Design review of the part built by this model. Coordinates are the model's own, in mm. A direction names the side the tool comes from. Give positions to 0.01 mm unless a question says otherwise; leave off trailing zeros. Loops run counter-clockwise (first coordinate to the right, second up) from the corner with the lowest first, then second, coordinate; pieces in that order, holes last. Notation, with made-up numbers: (70.25, -30.75) - (125.25, -30.75) arc R24 cw to (125.25, -11.75) - close; hole circle Ø6 at (53.25, 10). An arc over 180 degrees is marked (long way). Put each result on its own line as item: value. Start each with the question number.
```python
from build123d import *

# Parameters (mm, degrees)
F0_W     = 4
F0_H     = 4
F1_DEPTH = 55
F2_R     = 2
F3_DEPTH = 4
F4_R     = 2
F5_DEPTH = 4


with BuildPart() as f1:
    # F0 (on Front) → F1 (new body)
    with BuildSketch(Plane.XZ):
        Rectangle(F0_W, F0_H)
    extrude(amount=F1_DEPTH)

    # F2 (on face) → F3 (join)
    with BuildSketch(Plane(origin=(0, 0, 0), x_dir=(-1, 0, 0), z_dir=(0, 1, 0))):
        Circle(F2_R)
    extrude(amount=F3_DEPTH)

    # F4 (on face) → F5 (join)
    with BuildSketch(Plane.XZ.offset(55)):
        Circle(F4_R)
    extrude(amount=F5_DEPTH)


solid = f1.part
```
Item 1: For L1, parallel to X at y = -56, z = -0.2; L2, parallel to Z at x = 0.45, y = -55.5; L3, parallel to Y at x = -1.7, z = -1.6, list the stretches that pass through material, from the lowest coordinate up. Write a range as from..to.
Item 2: Consider section B-B (z = 1.4). State the section outline as (x, y) points, plus the area to 3 significant figures.
Item 3: Consider section A-A (x = 1.05). State the section outline as (y, z) points, plus the area to 3 significant figures.
Item 4: Machinability: for faces 1 (the flat face through (1.5, 0, 1.6)), 2 (the cylindrical face through (0, -57, -2)), 3 (the flat face through (-1.6, 0, -1.5)), 4 (the flat face through (-1.6, -55, 1.5)), which of the approach directions +Z, -Z, +X, -X, +Y, -Y give a long, thin tool a straight path to every point of the face, cutting with its end or side? Answer none if there is none.
Geometry says:
1. L1: x = -1.99..1.99
1. L2: z = -1.95..1.95
1. L3: y = -55..0
2. outline: (-2, -55) - (-1.43, -55) - (-1.43, -59) - (1.43, -59) - (1.43, -55) - (2, -55) - (2, 0) - (1.43, 0) - (1.43, 4) - (-1.43, 4) - (-1.43, 0) - (-2, 0) - close
2. area: 243 mm2
3. outline: (-59, -1.7) - (-55, -1.7) - (-55, -2) - (0, -2) - (0, -1.7) - (4, -1.7) - (4, 1.7) - (0, 1.7) - (0, 2) - (-55, 2) - (-55, 1.7) - (-59, 1.7) - close
3. area: 247 mm2
4. face 1: +Z, +X, +Y
4. face 2: -Y
4. face 3: -Z, -X, +Y
4. face 4: +Z, -X, -Y
